The model under review builds one solid part; all positions refer to its coordinate system, in mm. Round coordinates to 2 decimals unless told otherwise and drop trailing zeros. Write each loop counter-clockwise with the first axis right and the second up, starting at its lowest first coordinate (ties: lowest second). Pieces come first, ordered by that corner, then holes. Notation, with made-up numbers: M -8,1 L 2,1 A27 cw 2,38 Z; hole C 18.5,69 d7. An arc over 180 degrees is marked long. One line per item, written item: value. Start each with the question number.
1) Take a section at A-A, the plane y = 1.55. Write out the cut boundary in (x, z), and give its area (3 significant figures).
2) Take a section at C-C, the plane x = 5.5. Write out the cut boundary in (y, z), and give its area (3 significant figures).
3) Wall thickness on probe 1 along X at (y, z) = (0.3, -32); probe 2 along Z at (x, y) = (2, 1.9); probe 3 along Z at (x, y) = (4.25, 0.45): over which ranges is each line inside the solid? List them lowest first.
4) For P1, Ø6, axis at x = 4.5, z = -50.5, coming from the -Y side; P2, Ø1.5, axis at y = 1.5, z = -42.5, coming from the -X side; P3, Ø1.5, axis at x = 2.5, y = 2, coming from the +Z side, all flat-tipped, find the tip position at first contact; note any pin that passes through.
5) Take a section at B-B, the plane z = -12. Write out the cut boundary in (x, y), and give its area (3 significant figures).
6) Take a section at D-D, the plane z = -41.5. Write out the cut boundary in (x, y).
from build123d import *

# Parameters (mm, degrees)
EXTRUDE_1_DEPTH = 3
SKETCH_2_W      = 3.288983057
SKETCH_2_H      = 6.272081599
EXTRUDE_2_DEPTH = 3
SKETCH_3_W      = 10.5
SKETCH_3_H      = 28.238150406
EXTRUDE_3_DEPTH = 3


with BuildPart() as part:
    # 草图1 → 凸台-拉伸1 (new body)
    with BuildSketch(Plane(origin=(0, 0, 0), x_dir=(1, 0, 0), z_dir=(0, 1, 0))):
        with BuildLine():
            ThreePointArc((0, 14.5), (5.711829829, 13.327602935), (10.5, 10))
            Line((10.5, 10), (10.5, 31.761849594))
            Line((10.5, 31.761849594), (0, 31.761849594))
            Line((0, 31.761849594), (0, 14.5))
        make_face()
    extrude(amount=EXTRUDE_1_DEPTH)

    # 草图2 → 凸台-拉伸2 (add)
    with BuildSketch(Plane(origin=(0, 3, 0), x_dir=(1, 0, 0), z_dir=(0, 1, 0))):
        Polygon((-0.2, 14.5), (0, 14.5), (0, 24.347174928), (-3.488983057, 14.5), align=None)
        with Locations((-1.844491529, 11.363959201)):
            Rectangle(SKETCH_2_W, SKETCH_2_H)
    extrude(amount=-EXTRUDE_2_DEPTH)

    # 草图3 → 凸台-拉伸3 (add)
    with BuildSketch(Plane(origin=(0, 3, 0), x_dir=(1, 0, 0), z_dir=(0, 1, 0))):
        with Locations((5.25, 45.880924797)):
            Rectangle(SKETCH_3_W, SKETCH_3_H)
    extrude(amount=-EXTRUDE_3_DEPTH)


solid = part.part
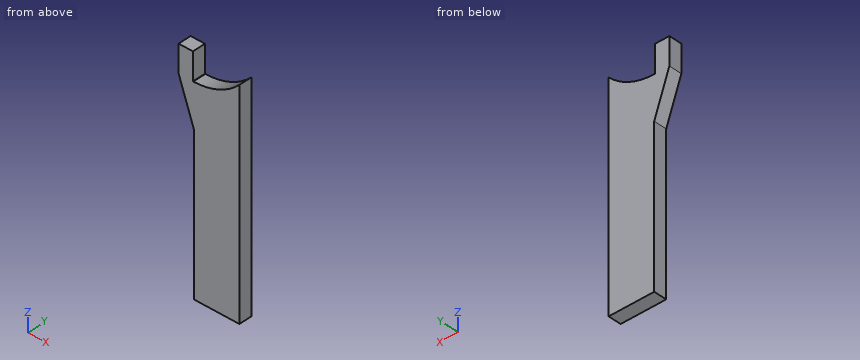
Checked values:
1. outline: M -3.49,-14.5 L 0,-24.35 L 0,-60 L 10.5,-60 L 10.5,-10 A14.5 cw 0,-14.5 L -0.2,-14.5 L -0.2,-8.23 L -3.49,-8.23 Z
1. area: 530 mm2
2. outline: M 0,-60 L 3,-60 L 3,-13.42 L 0,-13.42 Z
2. area: 140 mm2
3. probe 1: x = 0 to 10.5
3. probe 2: z = -60 to -14.36
3. probe 3: z = -60 to -13.86
4. P1: stops at y = 0
4. P2: stops at x = 0
4. P3: stops at z = -14.13
5. outline: M -3.49,0 L -0.2,0 L -0.2,3 L -3.49,3 Z; M 8.14,0 L 10.5,0 L 10.5,3 L 8.14,3 Z
5. area: 16.9 mm2
6. outline: M 0,0 L 10.5,0 L 10.5,3 L 0,3 Z
